from build123d import *

# Parameters (mm, degrees)
SKETCH1_R           = 10
BOSS_EXTRUDE1_DEPTH = 100
SKETCH2_R           = 5
CUT_EXTRUDE1_DEPTH  = 20
SKETCH3_R           = 3
CUT_EXTRUDE2_DEPTH  = 18


with BuildPart() as part:
    # Sketch1 → Boss-Extrude1 (new body)
    with BuildSketch(Plane(origin=(0, 0, 0), x_dir=(1, 0, 0), z_dir=(0, 1, 0))):
        Circle(SKETCH1_R)
    extrude(amount=BOSS_EXTRUDE1_DEPTH)

    # Sketch2 → Cut-Extrude1 (cut)
    with BuildSketch(Plane(origin=(0, 100, 0), x_dir=(1, 0, 0), z_dir=(0, 1, 0))):
        Circle(SKETCH2_R)
    extrude(amount=-CUT_EXTRUDE1_DEPTH, mode=Mode.SUBTRACT)

    # Sketch3 → Cut-Extrude2 (cut)
    with BuildSketch(Plane.XY):
        with Locations((0, 95)):
            Circle(SKETCH3_R)
    extrude(amount=-CUT_EXTRUDE2_DEPTH, mode=Mode.SUBTRACT)


solid = part.part
Model file for the job. Use its own axes, mm. A direction names the side the tool comes from. Round coordinates to 2 decimals unless told otherwise and drop trailing zeros. Order: outer loops, then holes, each group sorted by start corner. A loop starts at its lowest first (then second) coordinate and runs counter-clockwise, first axis right, second up.
(1) Band-saw the part on C-C (z = -7.25). List the corners of the cut face in (x, y), then the cut area to 3 significant figures.
(2) Drill centre lines: line 1 (Y direction, x = 0, z = -7.25); line 2 (Z direction, x = 0, y = 90). Where is each one in solid material? Low to high.
(3) 3-axis set-ups, long thin cutter, end or side, ignore diameter. For faces 1 (the face through (0, 0, 0)), 2 (the face through (-1.08, 90.14, 4.88)): which of +Z, -Z, +X, -X, +Y, -Y reach the whole face in a straight line?
(4) Band-saw the part on A-A (x = 0). List the corners of the cut face in (y, z).
(5) Pull direction Z, two halves, no side cores. Call faces 3 (the face through (0, 80, 0)), 4 (the face through (-2.17, 49.3, 9.76)), 5 (the face through (-0.65, 92.07, -6.97)): released by +Z, released by -Z, zero draft, split by the parting line, or undercut.
(6) Band-saw the part on B-B (z = 0). List the corners of the cut face in (x, y), then the cut area to 3 significant figures.
(7) Pin check, flat tips, straight feed: pin 1 (2 mm diameter, centred on x = 1.5, y = 58.5, fed in from -Z); pin 2 (2 mm diameter, centred on y = 72.5, z = -6.5, fed in from -X); pin 3 (4 mm diameter, centred on y = 60.5, z = 8, fed in from +X). Stop position of each tip, or through.
(8) Band-saw the part on D-D (y = 70.5). List the corners of the cut face in (x, z), then the cut area to 3 significant figures.
Verdict:
1. outline: (-6.89, 0) - (6.89, 0) - (6.89, 100) - (-6.89, 100) - close; hole circle Ø6 at (0, 95)
1. area: 1,350 mm2
2. line 1: y = 0 to 92, 98 to 100
2. line 2: z = -10 to -5, 5 to 10
3. face 1: +Z, -Z, +X, -X, -Y
3. face 2: +Y
4. outline: (0, -10) - (92, -10) - (92, -5) - (80, -5) - (80, 5) - (100, 5) - (100, 10) - (0, 10) - close; (98, -10) - (100, -10) - (100, -5) - (98, -5) - close
5. face 3: undercut
5. face 4: split by the parting line
5. face 5: zero draft
6. outline: (-10, 0) - (10, 0) - (10, 100) - (5, 100) - (5, 80) - (-5, 80) - (-5, 100) - (-10, 100) - close
6. area: 1,800 mm2
7. pin 1: stops at z = -9.99
7. pin 2: stops at x = -8.35
7. pin 3: stops at x = 8
8. outline: circle Ø20 at (0, 0)
8. area: 314 mm2
